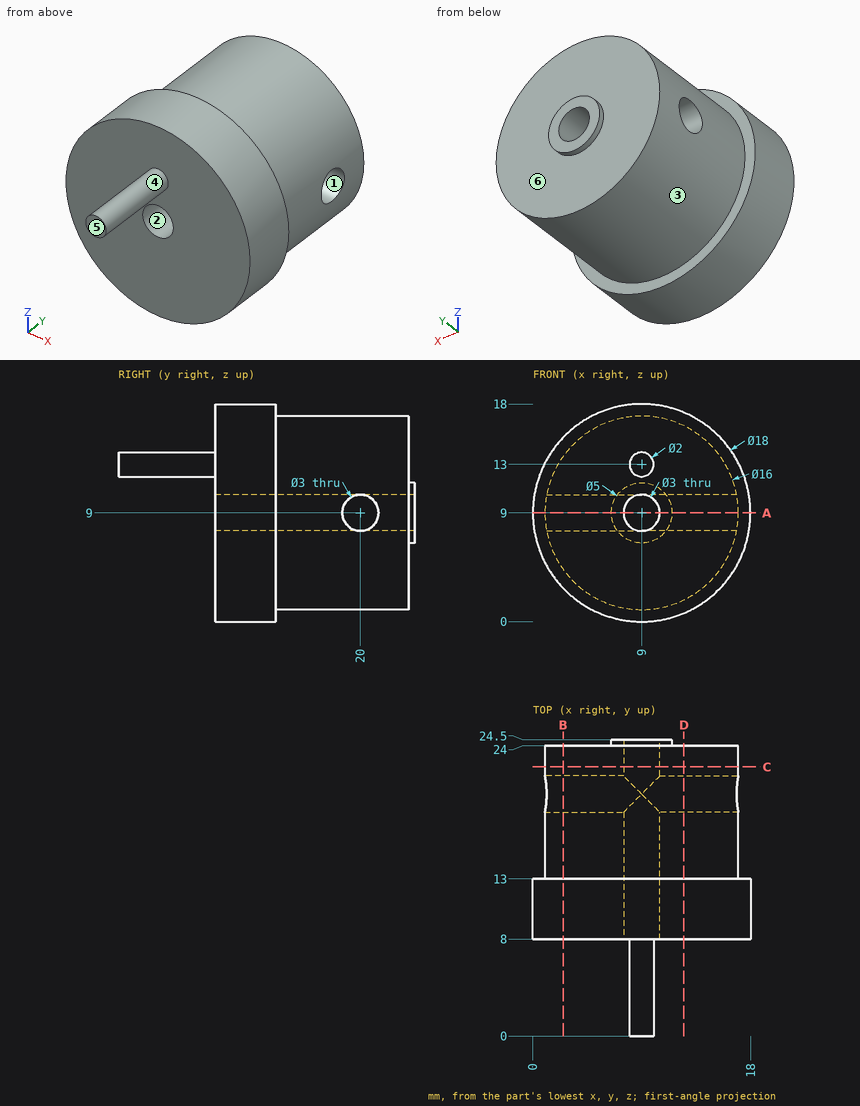
Geometry check sheet. Reference: drawing and pictorial views, mm from the part's lowest x, y, z. A direction names the side the tool comes from. Coordinates: 2 decimals unless noted, no trailing zeros. Order: outer loops, then holes, each group sorted by start corner. A loop starts at its lowest first (then second) coordinate and runs counter-clockwise, first axis right, second up. Notation, with made-up numbers: (-38.75, -3.5) - (-18.75, -3.5) arc R25 ccw to (-18.75, 11.5) - close; hole circle Ø9 at (14.25, 28). An arc over 180 degrees is marked (long way). One line per item, written item: value.
(1) Sectioned sample at D-D (x = 12.5). Enter the section's corners in (y, z), and give its area (3 significant figures).
Data:
outline: (8, 0.71) - (13, 0.71) - (13, 1.81) - (24, 1.81) - (24, 16.19) - (13, 16.19) - (13, 17.29) - (8, 17.29) - close; hole circle Ø3 at (20, 9)
area: 234 mm^2
(2) Sectioned sample at C-C (y = 22.25). Enter the section's corners in (x, z).
Data:
outline: circle Ø16 at (9, 9); hole circle Ø3 at (9, 9)
(3) Sectioned sample at A-A (z = 9). Enter the section's corners in (x, y).
Data:
outline: (0, 8) - (7.5, 8) - (7.5, 18.5) - (1, 18.5) - (1, 13) - (0, 13) - close; (1, 21.5) - (7.5, 21.5) - (7.5, 24.5) - (6.5, 24.5) - (6.5, 24) - (1, 24) - close; (10.5, 8) - (18, 8) - (18, 13) - (17, 13) - (17, 18.5) - (10.5, 18.5) - close; (10.5, 21.5) - (17, 21.5) - (17, 24) - (11.5, 24) - (11.5, 24.5) - (10.5, 24.5) - close
(4) Depth check by flat-ended pin: pin 1 Ø2.5 at (x, z) = (9, 9) entering from -Y; pin 2 Ø8 at (y, z) = (18.5, 13) entering from +X; pin 3 Ø3 at (y, z) = (9.5, 15) entering from +X; pin 4 Ø5 at (y, z) = (20, 9) entering from -X. Enter the tip coordinate at first touch or a pass-through.
Data:
pin 1: passes through
pin 2: stops at x = 17
pin 3: stops at x = 16.79
pin 4: stops at x = 1
(5) Thickness scan on probe 1 along Y at (x, z) = (14, 9); probe 2 along X at (y, z) = (21.9, 9). Record the ranges inside material, lowest first. Write a range as from..to.
Data:
probe 1: y = 8..18.5, 21.5..24
probe 2: x = 1..7.5, 10.5..17
(6) Release check for a two-part mould opening along X. For the marked faces 1, 2 and 3 record: +X half, -X half, draft (parallel to the pull), parting line (faces both ways), or undercut.
Data:
face 1: draft
face 2: undercut
face 3: parting line
(7) Access from +Z, -Z, +X, -X, +Y, -Y to the whole of each face (thin tool, end or side, straight path). Record for the marked faces 4, 5 and 6.
Data:
face 4: -Y
face 5: +Z, -Z, +X, -X, -Y
face 6: +Y
(8) Sectioned sample at B-B (x = 2.5). Enter the section's corners in (y, z), and give its area (3 significant figures).
Data:
outline: (8, 2.78) - (13, 2.78) - (13, 4.34) - (24, 4.34) - (24, 13.66) - (13, 13.66) - (13, 15.22) - (8, 15.22) - close; hole circle Ø3 at (20, 9)
area: 158 mm^2
